```python
from build123d import *

# Parameters (mm, degrees)
SKETCH1_R           = 25.4
BOSS_EXTRUDE1_DEPTH = 25.4
SKETCH2_R           = 38.1
SKETCH2_R_2         = 19.05
BOSS_EXTRUDE2_DEPTH = 12.7
SKETCH3_R           = 25.4
SKETCH3_R_2         = 19.05
CUT_EXTRUDE1_DEPTH  = 12.7
SKETCH5_R           = 39.751
SKETCH5_R_2         = 38.1
BOSS_EXTRUDE3_DEPTH = 2.54
SKETCH6_R           = 38.1
SKETCH6_R_2         = 36.449
CUT_EXTRUDE3_DEPTH  = 2.54


with BuildPart() as part:
    # Sketch1 → Boss-Extrude1 (new body)
    with BuildSketch(Plane(origin=(0, 0, 0), x_dir=(0, 0, -1), z_dir=(1, 0, 0))):
        Circle(SKETCH1_R)
        with BuildLine():
            Line((-2.38125, 10.854368), (-2.38125, 13.49375))
            Line((-2.38125, 13.49375), (2.38125, 13.49375))
            Line((2.38125, 13.49375), (2.38125, 10.854368))
            ThreePointArc((2.38125, 10.854368), (8.658790241, 6.965127982), (11.1125, 0))
            ThreePointArc((11.1125, 0), (-6.965127982, -8.658790241), (-2.38125, 10.854368))
        make_face(mode=Mode.SUBTRACT)
    extrude(amount=BOSS_EXTRUDE1_DEPTH)

    # Sketch2 → Boss-Extrude2 (add)
    with BuildSketch(Plane.ZY):
        Circle(SKETCH2_R)
        Circle(SKETCH2_R_2, mode=Mode.SUBTRACT)
    extrude(amount=-BOSS_EXTRUDE2_DEPTH)

    # Sketch3 → Cut-Extrude1 (cut)
    with BuildSketch(Plane(origin=(25.4, 0, 0), x_dir=(0, 0, -1), z_dir=(1, 0, 0))):
        Circle(SKETCH3_R)
        Circle(SKETCH3_R_2, mode=Mode.SUBTRACT)
    extrude(amount=-CUT_EXTRUDE1_DEPTH, mode=Mode.SUBTRACT)

    # Sketch5 → Boss-Extrude3 (add)
    with BuildSketch(Plane.ZY):
        Circle(SKETCH5_R)
        Circle(SKETCH5_R_2, mode=Mode.SUBTRACT)
    extrude(amount=-BOSS_EXTRUDE3_DEPTH)

    # Sketch6 → Cut-Extrude3 (cut)
    with BuildSketch(Plane(origin=(12.7, 0, 0), x_dir=(0, 0, -1), z_dir=(1, 0, 0))):
        Circle(SKETCH6_R)
        Circle(SKETCH6_R_2, mode=Mode.SUBTRACT)
    extrude(amount=-CUT_EXTRUDE3_DEPTH, mode=Mode.SUBTRACT)


solid = part.part
```
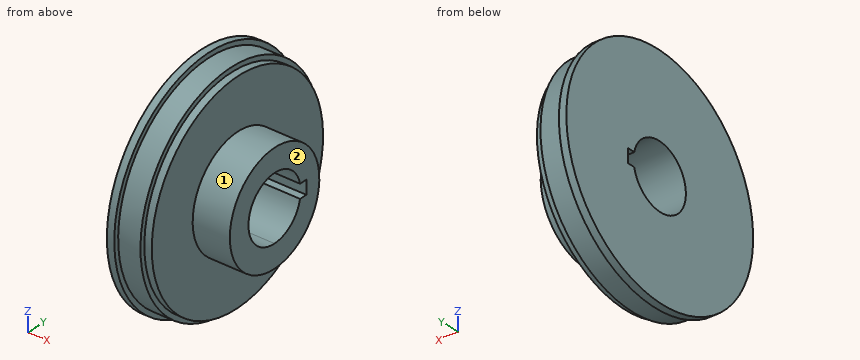
Model file for the job. Use its own axes, mm. Face numbers are marked on the shaded views. A direction names the side the tool comes from. Give positions to 0.01 mm unless a question says otherwise; leave off trailing zeros. Write each loop counter-clockwise with the first axis right and the second up, starting at its lowest first coordinate (ties: lowest second). Pieces come first, ordered by that corner, then holes. Notation, with made-up numbers: (28, 6.25) - (55, 6.25) arc R35 cw to (55, 42.25) - close; hole circle Ø9 at (7, -16). An arc over 180 degrees is marked (long way). One line per question, with ' | ' between items. Start each with the question number.
(1) Pin check, flat tips, straight feed: P1, Ø1.3, axis at x = 14.5, y = 12.5, coming from the +Z side; P2, Ø12, axis at x = 12, z = 16.5, coming from the -Y side; P3, Ø1.3, axis at x = 15, y = 12.5, coming from the -Z side. Stop position of each tip, or through.
(2) Wall check: line 1 along Y through (x, z) = (9.75, 0); line 2 along Y through (x, z) = (14, 0); line 3 along Z through (x, y) = (16.75, 7). Give the ranges that are in metal, low to high. Write a range as from..to.
(3) Slice it at A-A on z = 0. Write the cut outline in (x, y), plus the area to 3 significant figures.
(4) 3-axis set-ups, long thin cutter, end or side, ignore diameter. For the marked faces 1 and 2: which of +Z, -Z, +X, -X, +Y, -Y reach the whole face in a straight line?
(5) Slice it at D-D on y = 30. Write the cut outline in (x, z).
(6) Slice it at C-C on y = 1. Write the cut outline in (x, z).
Results below:
1) P1: z = 14.92 | P2: y = -36.54 | P3: z = -14.92
2) line 1: -38.1..-11.11, 13.49..38.1 | line 2: -19.05..-11.11, 13.49..19.05 | line 3: -17.72..-8.63, 8.63..17.72
3) outline: (0, -39.75) - (2.54, -39.75) - (2.54, -38.1) - (10.16, -38.1) - (10.16, -36.45) - (12.7, -36.45) - (12.7, -19.05) - (25.4, -19.05) - (25.4, -11.11) - (0, -11.11) - close; (0, 13.49) - (25.4, 13.49) - (25.4, 19.05) - (12.7, 19.05) - (12.7, 36.45) - (10.16, 36.45) - (10.16, 38.1) - (2.54, 38.1) - (2.54, 39.75) - (0, 39.75) - close | area: 827 mm^2
4) face 1: +X | face 2: +Z, -Z, +X, +Y, -Y
5) outline: (0, -26.08) - (2.54, -26.08) - (2.54, -23.49) - (10.16, -23.49) - (10.16, -20.7) - (12.7, -20.7) - (12.7, 20.7) - (10.16, 20.7) - (10.16, 23.49) - (2.54, 23.49) - (2.54, 26.08) - (0, 26.08) - close
6) outline: (0, -39.74) - (2.54, -39.74) - (2.54, -38.09) - (10.16, -38.09) - (10.16, -36.44) - (12.7, -36.44) - (12.7, -19.02) - (25.4, -19.02) - (25.4, -11.07) - (0, -11.07) - close; (0, 11.07) - (25.4, 11.07) - (25.4, 19.02) - (12.7, 19.02) - (12.7, 36.44) - (10.16, 36.44) - (10.16, 38.09) - (2.54, 38.09) - (2.54, 39.74) - (0, 39.74) - close
